from build123d import *

# Parameters (mm, degrees)
F0_W     = 100
F0_H     = 100
F1_DEPTH = 100
F2_W     = 100
F2_H     = 70
F3_DEPTH = 42
F4_W     = 60
F4_H     = 20
F5_DEPTH = 25


with BuildPart() as f1:
    # F0 (on Top) → F1 (new body)
    with BuildSketch(Plane.XY):
        Rectangle(F0_W, F0_H)
    extrude(amount=F1_DEPTH)

    # F2 (on face) → F3 (cut)
    with BuildSketch(Plane.XY.offset(100)):
        with Locations((0, -15)):
            Rectangle(F2_W, F2_H)
    extrude(amount=-F3_DEPTH, mode=Mode.SUBTRACT)

    # F4 (on face) → F5 (cut)
    with BuildSketch(Plane.XZ.offset(50)):
        with Locations((-2.848295, 10)):
            Rectangle(F4_W, F4_H)
    extrude(amount=-F5_DEPTH, mode=Mode.SUBTRACT)


solid = f1.part
Could you check a few things on this model? Use its own coordinates, in mm. A direction names the side the tool comes from. Give positions to 0.01 mm unless a question says otherwise; leave off trailing zeros. Order: outer loops, then holes, each group sorted by start corner. A loop starts at its lowest first (then second) coordinate and runs counter-clockwise, first axis right, second up.
1. Suppose I cut it at A-A (x = -3). Write out the boundary of the cut face in (y, z).
Answers below:
outline: (-50, 20) - (-25, 20) - (-25, 0) - (50, 0) - (50, 100) - (20, 100) - (20, 58) - (-50, 58) - close
2. Suppose I cut it at D-D (z = 70). Write out the boundary of the cut face in (x, y), plus the area to 3 significant figures.
Answers below:
outline: (-50, 20) - (50, 20) - (50, 50) - (-50, 50) - close
area: 3,000 mm2
3. I need wall thicknesses on L1, parallel to Y at x = 0.5, z = 70; L2, parallel to Z at x = -5, y = 5; L3, parallel to Z at x = -11, y = -37. Which ranges of each line are inside material? Lowest first, please.
Answers below:
L1: y = 20 to 50
L2: z = 0 to 58
L3: z = 20 to 58
4. Suppose I cut it at C-C (y = 1). Write out the boundary of the cut face in (x, z), plus the area to 3 significant figures.
Answers below:
outline: (-50, 0) - (50, 0) - (50, 58) - (-50, 58) - close
area: 5,800 mm2
5. Which directions (+Z, -Z, +X, -X, +Y, -Y) give clear straight access to the entire face, cutting with the end or side of a thin tool? Please do faces 4 (the flat face through (-1, 20, 79)), 5 (the flat face through (-1, 35, 100)), 6 (the flat face through (-32.848, -38, 10)).
Answers below:
face 4: +Z, +X, -X, -Y
face 5: +Z, +X, -X, +Y, -Y
face 6: -Z, -Y
6. Suppose I cut it at B-B (z = 9.5). Write out the boundary of the cut face in (x, y).
Answers below:
outline: (-50, -50) - (-32.85, -50) - (-32.85, -25) - (27.15, -25) - (27.15, -50) - (50, -50) - (50, 50) - (-50, 50) - close
7. For pin 1 (1 mm diameter, centred on x = -3, y = -31, fed in from +Z); pin 2 (6 mm diameter, centred on x = 4, z = 12, fed in from -Y); pin 3 (7.5 mm diameter, centred on x = -4, y = -33.5, fed in from -Z), each with a flat end and sliding along its axis, tell me the tip position at first contact or that it passes through.
Answers below:
pin 1: stops at z = 58
pin 2: stops at y = -25
pin 3: stops at z = 20
8. Thinking about a two-plate mould opening in X: for faces 1 (the flat face through (-50, 10, 38)), 2 (the flat face through (-1, 50, 49)), 3 (the flat face through (-3, -38, 20)), which applies, +X half, -X half, draft (parallel to the pull), parting line (faces both ways), or undercut?
Answers below:
face 1: -X half
face 2: draft
face 3: undercut
